Job drawing, mm, ordinate dimensions from the low corner. One solid piece. A direction names the side the tool comes from. Give positions to 0.01 mm unless a question says otherwise; leave off trailing zeros. Order: outer loops, then holes, each group sorted by start corner. A loop starts at its lowest first (then second) coordinate and runs counter-clockwise, first axis right, second up. Notation, with made-up numbers: M -11.75,4 L 7.25,4 A23 cw 7.25,24 Z; hole C -1.75,-34 d2. An arc over 180 degrees is marked long. Put each result on its own line as item: value. Start each with the question number.
1) Cut at C-C (z = 15.25). Write the cut outline in (x, y) (3 decimals).
2) Cut at A-A (y = 25.4). Write the cut outline in (x, z) (3 decimals).
3) Two-plate mould, pull along Y, no slides. Class the marked faces 1, 2 and 3: released by +Y, released by -Y, zero draft, split by the parting line, or undercut.
4) Cut at D-D (y = 6). Write the cut outline in (x, z), and give its area (3 significant figures).
5) Drill centre lines: line 1 (X direction, y = 4.5, z = 11.5); line 2 (X direction, y = 4, z = 17.75); line 3 (Y direction, x = 45, z = 1). Where is each one in solid material? Low to high. Write a range as [from, to].
6) Pin check, flat tips, straight feed: pin 1 (3.5 mm diameter, centred on x = 46.355, y = 46.355, fed in from +Z); pin 2 (3 mm diameter, centred on y = 23.5, z = 15, fed in from -X) (3 decimals); pin 3 (6.5 mm diameter, centred on y = 26, z = 10.5, fed in from +X) (3 decimals); pin 4 (6.5 mm diameter, centred on x = 25.5, z = 8, fed in from -Y) (3 decimals). Stop position of each tip, or through.
7) Tool access for the marked faces 4, 5, 6, 7 and 8: list every direction of +Z, -Z, +X, -X, +Y, -Y with a clear straight run to the whole face (end or side of a thin tool).
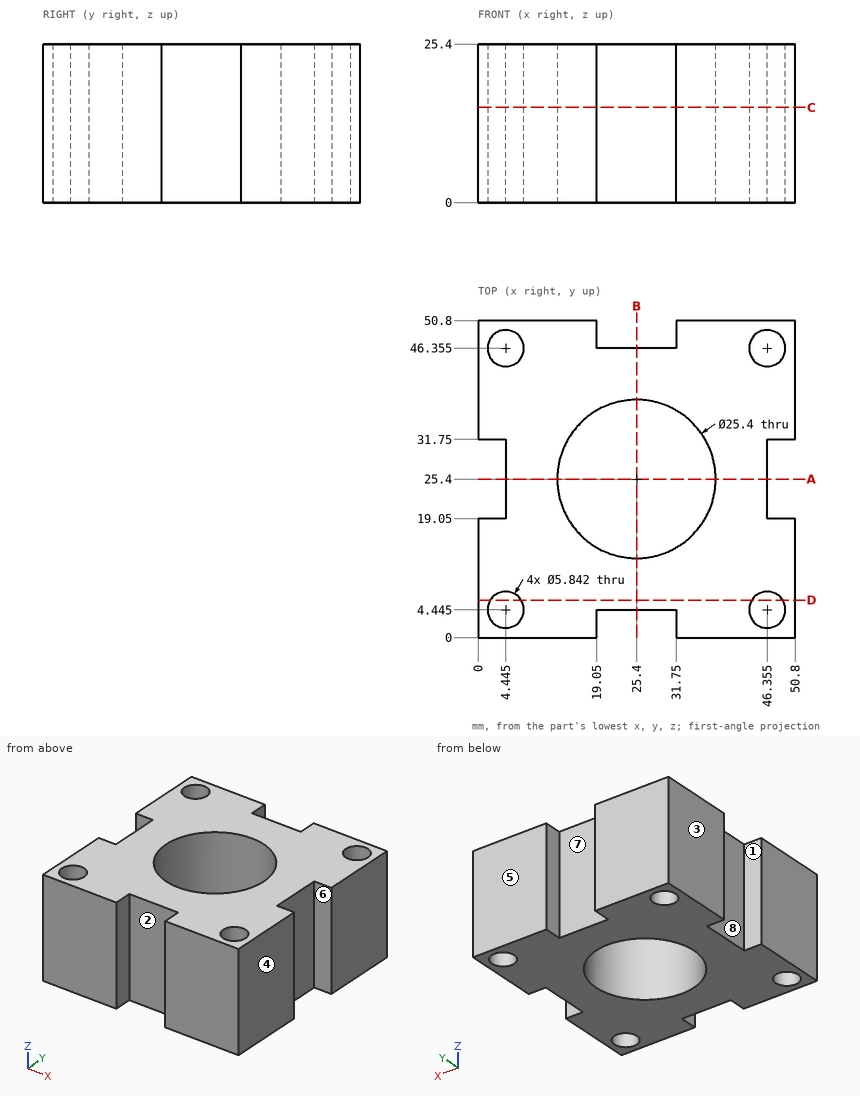
Solution:
1. outline: M 0,0 L 19.05,0 L 19.05,4.445 L 31.75,4.445 L 31.75,0 L 50.8,0 L 50.8,19.05 L 46.355,19.05 L 46.355,31.75 L 50.8,31.75 L 50.8,50.8 L 31.75,50.8 L 31.75,46.355 L 19.05,46.355 L 19.05,50.8 L 0,50.8 L 0,31.75 L 4.445,31.75 L 4.445,19.05 L 0,19.05 Z; hole C 4.445,4.445 d5.842; hole C 4.445,46.355 d5.842; hole C 25.4,25.4 d25.4; hole C 46.355,4.445 d5.842; hole C 46.355,46.355 d5.842
2. outline: M 4.445,0 L 12.7,0 L 12.7,25.4 L 4.445,25.4 Z; M 38.1,0 L 46.355,0 L 46.355,25.4 L 38.1,25.4 Z
3. face 1: undercut
3. face 2: released by -Y
3. face 3: zero draft
4. outline: M 0,0 L 1.97,0 L 1.97,25.4 L 0,25.4 Z; M 6.92,0 L 43.88,0 L 43.88,25.4 L 6.92,25.4 Z; M 48.83,0 L 50.8,0 L 50.8,25.4 L 48.83,25.4 Z
4. area: 1,040 mm²
5. line 1: [0, 1.52], [7.37, 43.43], [49.28, 50.8]
5. line 2: [0, 1.56], [7.33, 19.05], [31.75, 43.47], [49.24, 50.8]
5. line 3: [0, 1.86], [7.03, 43.77], [48.94, 50.8]
6. pin 1: through
6. pin 2: x = 4.445
6. pin 3: x = 46.355
6. pin 4: y = 4.445
7. face 4: +Z, -Z, +X, +Y, -Y
7. face 5: +Z, -Z, +X, -X, +Y
7. face 6: +Z, -Z, +X
7. face 7: +Z, -Z, +Y
7. face 8: +Z, -Z, -X
